from build123d import *

# Parameters (mm, degrees)
BOSS_EXTRUDE1_DEPTH = 40
SKETCH2_R           = 70
CUT_EXTRUDE1_DEPTH  = 15
SKETCH3_R           = 64
SKETCH3_R_2         = 49
CUT_EXTRUDE3_DEPTH  = 8
SKETCH4_R           = 4.75
CUT_EXTRUDE4_DEPTH  = 18
SKETCH5_R           = 25
CUT_EXTRUDE5_DEPTH  = 26
SKETCH7_R           = 43
CUT_EXTRUDE6_DEPTH  = 15
CUT_EXTRUDE7_DEPTH  = 38.5
SKETCH9_R           = 13.664776458
SKETCH9_R_2         = 7.722805547
CUT_EXTRUDE8_DEPTH  = 41
FILLET1_R           = 2
SKETCH10_W          = 4
SKETCH10_H          = 9
BOSS_EXTRUDE2_DEPTH = 1.5
SKETCH11_R          = 2
CUT_EXTRUDE9_DEPTH  = 4


with BuildPart() as part:
    # Sketch1 → Boss-Extrude1 (new body)
    with BuildSketch(Plane(origin=(0, 0, 0), x_dir=(1, 0, 0), z_dir=(0, 1, 0))):
        with BuildLine():
            Line((-257.832794656, 48.5), (-160, 48.5))
            Line((-160, 48.5), (-115.769532107, 68.397630762))
            ThreePointArc((-115.769532107, 68.397630762), (-10, 0), (-115.769532107, -68.397630762))
            Line((-115.769532107, -68.397630762), (-160, -48.5))
            Line((-160, -48.5), (-257.832794656, -48.5))
            ThreePointArc((-257.832794656, -48.5), (-267.732532415, -44.769214361), (-272.707763578, -35.432692308))
            ThreePointArc((-272.707763578, -35.432692308), (-275, 0), (-272.707763578, 35.432692308))
            ThreePointArc((-272.707763578, 35.432692308), (-267.732532415, 44.769214361), (-257.832794656, 48.5))
        make_face()
    extrude(amount=BOSS_EXTRUDE1_DEPTH)

    # Sketch2 → Cut-Extrude1 (cut)
    with BuildSketch(Plane(origin=(0, 40, 0), x_dir=(1, 0, 0), z_dir=(0, 1, 0))):
        with Locations((-85, 0)):
            Circle(SKETCH2_R)
    extrude(amount=-CUT_EXTRUDE1_DEPTH, mode=Mode.SUBTRACT)

    # Sketch3 → Cut-Extrude3 (cut)
    with BuildSketch(Plane(origin=(0, 25, 0), x_dir=(1, 0, 0), z_dir=(0, 1, 0))):
        with Locations((-85, 0)):
            Circle(SKETCH3_R)
        with Locations((-85, 0)):
            Circle(SKETCH3_R_2, mode=Mode.SUBTRACT)
    extrude(amount=-CUT_EXTRUDE3_DEPTH, mode=Mode.SUBTRACT)

    # Sketch4 → Cut-Extrude4 (cut, through all)
    with BuildSketch(Plane(origin=(0, 17, 0), x_dir=(1, 0, 0), z_dir=(0, 1, 0))):
        with Locations((-45.048466863, -39.951533137)):
            Circle(SKETCH4_R)
        with Locations((-85, -56.5)):
            Circle(SKETCH4_R)
        with Locations((-28.5, 0)):
            Circle(SKETCH4_R)
        with Locations((-124.951533137, -39.951533137)):
            Circle(SKETCH4_R)
        with Locations((-141.5, 0)):
            Circle(SKETCH4_R)
        with Locations((-124.951533137, 39.951533137)):
            Circle(SKETCH4_R)
        with Locations((-85, 56.5)):
            Circle(SKETCH4_R)
        with Locations((-45.048466863, 39.951533137)):
            Circle(SKETCH4_R)
    extrude(amount=-CUT_EXTRUDE4_DEPTH, mode=Mode.SUBTRACT)

    # Sketch5 → Cut-Extrude5 (cut, through all)
    with BuildSketch(Plane(origin=(0, 25, 0), x_dir=(1, 0, 0), z_dir=(0, 1, 0))):
        with Locations((-85, 0)):
            Circle(SKETCH5_R)
    extrude(amount=-CUT_EXTRUDE5_DEPTH, mode=Mode.SUBTRACT)

    # Sketch7 → Cut-Extrude6 (cut)
    with BuildSketch(Plane(origin=(0, 25, 0), x_dir=(1, 0, 0), z_dir=(0, 1, 0))):
        with Locations((-85, 0)):
            Circle(SKETCH7_R)
    extrude(amount=-CUT_EXTRUDE6_DEPTH, mode=Mode.SUBTRACT)

    # Sketch8 → Cut-Extrude7 (cut)
    with BuildSketch(Plane.XZ):
        with BuildLine():
            Line((-257.832794656, 45.5), (-160, 45.5))
            Line((-160, 45.5), (-160, -45.5))
            Line((-160, -45.5), (-257.832794656, -45.5))
            ThreePointArc((-257.832794656, -45.5), (-265.752584863, -42.515371489), (-269.732769794, -35.046153846))
            ThreePointArc((-269.732769794, -35.046153846), (-272, 0), (-269.732769794, 35.046153846))
            ThreePointArc((-269.732769794, 35.046153846), (-265.752584863, 42.515371489), (-257.832794656, 45.5))
        make_face()
    extrude(amount=-CUT_EXTRUDE7_DEPTH, mode=Mode.SUBTRACT)

    # Sketch9 → Cut-Extrude8 (cut, through all)
    with BuildSketch(Plane(origin=(0, 40, 0), x_dir=(1, 0, 0), z_dir=(0, 1, 0))):
        with Locations((-221.059573663, 22.236353901)):
            Circle(SKETCH9_R)
        with Locations((-209.874820802, -7.855957366)):
            Circle(SKETCH9_R_2)
    extrude(amount=-CUT_EXTRUDE8_DEPTH, mode=Mode.SUBTRACT)

    # Fillet1
    fillet1_edges = [part.edges().sort_by_distance(p)[0] for p in [
        (-267.732532415, 40, 44.769214361),
        (-208.916397328, 40, 48.5),
        (-208.916397328, 40, -48.5),
        (-267.732532415, 40, -44.769214361),
        (-275, 40, 0),
    ]]
    fillet(fillet1_edges, radius=FILLET1_R)

    # Sketch10 → Boss-Extrude2 (add)
    with BuildSketch(Plane.XY.offset(-45.5)):
        with Locations((-252.832794656, 0)):
            Rectangle(SKETCH10_W, SKETCH10_H)
        with Locations((-185.832794656, 0)):
            Rectangle(SKETCH10_W, SKETCH10_H)
    boss_extrude2 = extrude(amount=-BOSS_EXTRUDE2_DEPTH)

    # Mirror1: Boss-Extrude2 across plane
    add(boss_extrude2.mirror(Plane.XY))

    # Sketch11 → Cut-Extrude9 (cut)
    with BuildSketch(Plane.XZ):
        with Locations((-106, 21)):
            Circle(SKETCH11_R)
        with Locations((-64, 21)):
            Circle(SKETCH11_R)
        with Locations((-64, -21)):
            Circle(SKETCH11_R)
        with Locations((-106, -21)):
            Circle(SKETCH11_R)
    extrude(amount=-CUT_EXTRUDE9_DEPTH, mode=Mode.SUBTRACT)


solid = part.part
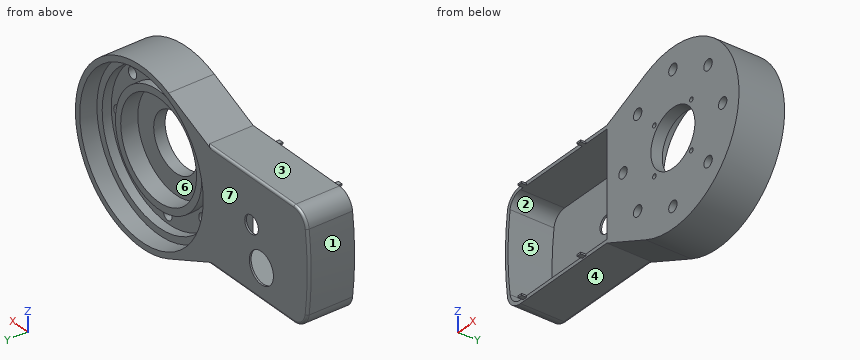
Read the model definition and answer for the solid it produces. Units are mm, in the model's axes. Face numbers are marked on the shaded views. A direction names the side the tool comes from. Round coordinates to 2 decimals unless told otherwise and drop trailing zeros. Write each loop counter-clockwise with the first axis right and the second up, starting at its lowest first coordinate (ties: lowest second). Pieces come first, ordered by that corner, then holes.
Q1. A tool of negligible diameter and unlimited length cuts with its end or side. For the marked faces 4, 5, 6 and 7, from which of +Z, -Z, +X, -X, +Y, -Y can it reach the whole face along a straight path? Write none if from no direction.
Values:
face 4: -Z, -X, +Y, -Y
face 5: -Y
face 6: +Y
face 7: +Z, -Z, +X, -X, +Y
Q2. Find section A-A on y = 35.5. Determine the outline of the cut face in (x, z).
Values:
outline: (-272.71, -35.43) arc R15 ccw to (-257.83, -48.5) - (-160, -48.5) - (-115.77, -68.4) arc R75 ccw (long way) to (-115.77, 68.4) - (-160, 48.5) - (-257.83, 48.5) arc R15 ccw to (-272.71, 35.43) arc R275 ccw to start; hole (-269.73, -35.05) arc R12 ccw to (-257.83, -45.5) - (-160, -45.5) - (-160, 45.5) - (-257.83, 45.5) arc R12 ccw to (-269.73, 35.05) arc R272 ccw to start; hole circle Ø140 at (-85, 0)
Q3. Find section B-B on z = -56.5. Determine the outline of the cut face in (x, y).
Values:
outline: (-142.22, 0) - (-89.75, 0) - (-89.75, 17) - (-115.06, 17) - (-115.06, 25) - (-126.32, 25) - (-126.32, 40) - (-142.22, 40) - close; (-80.25, 0) - (-35.68, 0) - (-35.68, 40) - (-43.68, 40) - (-43.68, 25) - (-54.94, 25) - (-54.94, 17) - (-80.25, 17) - close
Q4. Flat-ended cylindrical pins translate along their axes: P1, Ø6, axis at x = -166, z = 23.5, coming from the -Y side; P2, Ø2, axis at x = -47.5, z = -56, coming from the -Y side; P3, Ø3, axis at x = -106, z = 21, coming from the +Y side. Find the tip coordinate at first contact, or state that the pin passes through.
Values:
P1: stops at y = 38.5
P2: stops at y = 0
P3: stops at y = 10
Q5. The mould has two halves that part along X. Classify the marked faces 1, 2 and 3: released by +X, released by -X, zero draft, split by the parting line, or undercut.
Values:
face 1: released by -X
face 2: undercut
face 3: zero draft
Q6. Straight lines are drawn through the part: line 1 (Z direction, x = -86.5, y = 20) (3 decimals); line 2 (Z direction, x = -85, y = 7); line 3 (Z direction, x = -169, y = 29). For each, find the intervals that lie inside material, in ascending order.
Values:
line 1: z = -74.985 to -63.982, -48.977 to -42.974, 42.974 to 48.977, 63.982 to 74.985
line 2: z = -75 to -61.25, -51.75 to -25, 25 to 51.75, 61.25 to 75
line 3: z = -48.5 to -45.5, 45.5 to 48.5
Q7. Find section D-D on x = -55. Determine the outline of the cut face in (y, z), and give its area (3 significant figures).
Values:
outline: (0, -68.74) - (40, -68.74) - (40, -63.25) - (25, -63.25) - (25, -56.53) - (17, -56.53) - (17, -38.74) - (25, -38.74) - (25, -30.81) - (10, -30.81) - (10, 30.81) - (25, 30.81) - (25, 38.74) - (17, 38.74) - (17, 56.53) - (25, 56.53) - (25, 63.25) - (40, 63.25) - (40, 68.74) - (0, 68.74) - close
area: 2,390 mm2
Q8. Find section C-C on x = -141.5. Determine the outline of the cut face in (y, z), and give its area (3 significant figures).
Values:
outline: (0, -56.82) - (40, -56.82) - (40, -41.32) - (25, -41.32) - (25, -30.06) - (17, -30.06) - (17, -4.75) - (0, -4.75) - close; (0, 4.75) - (17, 4.75) - (17, 30.06) - (25, 30.06) - (25, 41.32) - (40, 41.32) - (40, 56.82) - (0, 56.82) - close
area: 2,660 mm2
